Answer from the drawing. Dimensions are ordinates in mm from the lowest x, y and z of the part. A direction names the side the tool comes from. Round coordinates to 2 decimals unless told otherwise and drop trailing zeros. Loops run counter-clockwise (first coordinate to the right, second up) from the corner with the lowest first, then second, coordinate; pieces in that order, holes last. Notation, with made-up numbers: (56.5, 70.5) - (97.5, 70.5) arc R11 cw to (97.5, 86.5) - close; hole circle Ø10 at (25, -10.5). An arc over 180 degrees is marked (long way). Answer as CSV lines item,"result".
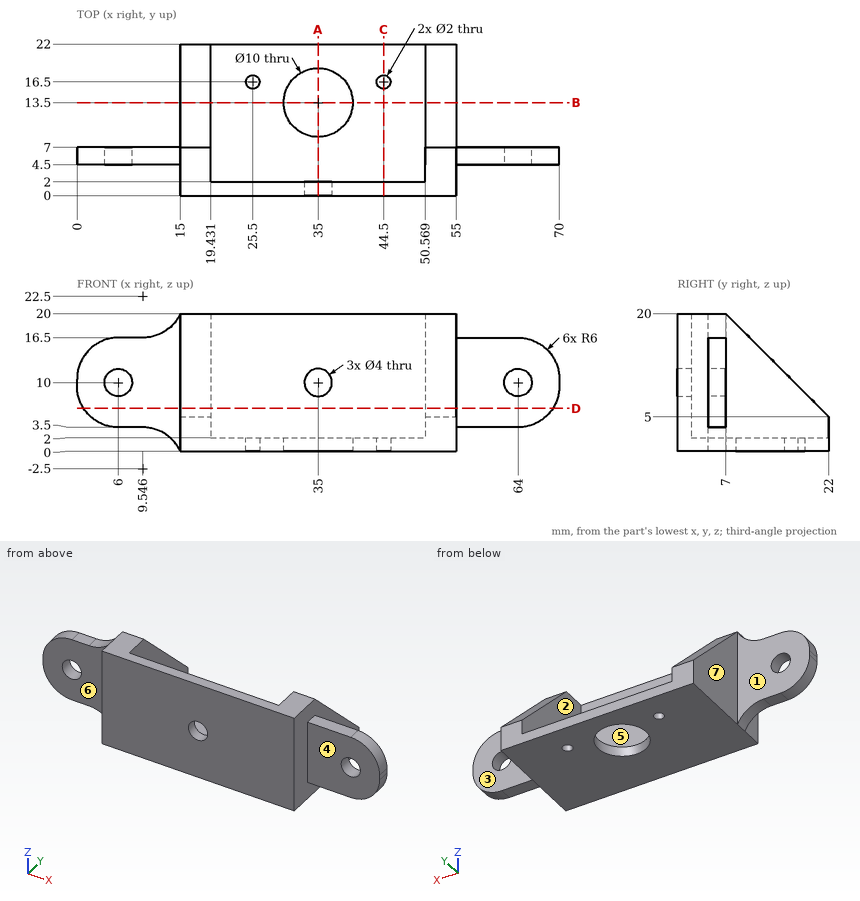
1) A cutting plane is placed at C-C, the plane x = 44.5. Determine the outline of the cut face in (y, z).
Entries:
outline,"(0, 0) - (15.5, 0) - (15.5, 2) - (2, 2) - (2, 20) - (0, 20) - close; (17.5, 0) - (22, 0) - (22, 2) - (17.5, 2) - close"
2) Each of these flat-tipped pins is pushed along its axis until it touches: P1, Ø5, axis at x = 6, z = 10, coming from the -Y side; P2, Ø3, axis at x = 8, y = 6, coming from the +Z side; P3, Ø2, axis at y = 2.5, z = 6, coming from the -X side. Where does it stop, or does it pass through?
Entries:
P1,"stops at y = 4.5"
P2,"stops at z = 16.5"
P3,"stops at x = 15"
3) A cutting plane is placed at D-D, the plane z = 6.25. Determine the outline of the cut face in (x, y).
Entries:
outline,"(0.96, 4.5) - (15, 4.5) - (15, 0) - (55, 0) - (55, 4.5) - (69.04, 4.5) - (69.04, 7) - (55, 7) - (55, 20.75) - (50.57, 20.75) - (50.57, 2) - (19.43, 2) - (19.43, 20.75) - (15, 20.75) - (15, 7) - (0.96, 7) - close"
4) A tool of negligible diameter and unlimited length cuts with its end or side. For the marked faces 1, 2, 3 and 4, from which of +Z, -Z, +X, -X, +Y, -Y can it reach the whole face along a straight path? Write none if from no direction.
Entries:
face 1,"+Z, -Z, -X, +Y"
face 2,"+Z, +Y"
face 3,"+Z, -Z, +X, +Y"
face 4,"+Z, -Z, +X, -Y"
5) Find the intervals of material crossed by line 1 (X direction, y = 14.5, z = 4.25); line 2 (Z direction, x = 64, y = 6.5); line 3 (Y direction, x = 35, z = 0.95), in increasing order.
Entries:
line 1,"x = 15 to 19.43, 50.57 to 55"
line 2,"z = 3.5 to 8, 12 to 16.5"
line 3,"y = 0 to 8.5, 18.5 to 22"
6) A cutting plane is placed at B-B, the plane y = 13.5. Determine the outline of the cut face in (x, z), plus the area to 3 significant figures.
Entries:
outline,"(15, 0) - (30, 0) - (30, 2) - (19.43, 2) - (19.43, 13.5) - (15, 13.5) - close; (40, 0) - (55, 0) - (55, 13.5) - (50.57, 13.5) - (50.57, 2) - (40, 2) - close"
area,"162 mm^2"
7) A cutting plane is placed at A-A, the plane x = 35. Determine the outline of the cut face in (y, z).
Entries:
outline,"(0, 0) - (8.5, 0) - (8.5, 2) - (2, 2) - (2, 8) - (0, 8) - close; (0, 12) - (2, 12) - (2, 20) - (0, 20) - close; (18.5, 0) - (22, 0) - (22, 2) - (18.5, 2) - close"
8) The mould has two halves that part along X. Classify the marked faces 5, 6 and 7: pulls with the +X half, pulls with the -X half, needs draft (parallel to the pull), parting line crosses it, or undercut.
Entries:
face 5,"undercut"
face 6,"needs draft"
face 7,"pulls with the -X half"
